Verification items for the finished model (mm, model axes). A direction names the side the tool comes from. Round coordinates to 2 decimals unless told otherwise and drop trailing zeros. Loops run counter-clockwise (first coordinate to the right, second up) from the corner with the lowest first, then second, coordinate; pieces in that order, holes last. Notation, with made-up numbers: M 61.5,44.25 L 76.5,44.25 A33 cw 76.5,72.25 Z; hole C 82.25,27 d10. An arc over 180 degrees is marked long. One line per item, written item: value.
Autodesk Inventor part; units mm, degrees
ref_plane "Work Plane1" through (0, 12.7, 0) normal (0, -1, 0) x (1, 0, 0)
ref_plane "YZ Plane" through (0, 0, 0) normal (1, 0, 0) x (0, 1, 0)
ref_plane "XZ Plane" through (0, 0, 0) normal (0, 1, 0) x (-1, 0, 0)
sketch "Sketch1" plane through (0, 0, 0) normal (0, 0, 1) x (1, 0, 0)
  line L0 (0, 0) -> (50.8, 0)
  line L1 (50.8, 0) -> (50.8, 25.4)
  line L2 (50.8, 25.4) -> (0, 25.4)
  line L3 (0, 25.4) -> (0, 0)
  line L4 (3.175, 22.225) -> (47.625, 22.225)
  line L5 (47.625, 22.225) -> (47.625, 3.175)
  line L6 (47.625, 3.175) -> (3.175, 3.175)
  line L7 (3.175, 3.175) -> (3.175, 22.225)
  dimension "d0" = 50.8
  dimension "d1" = 25.4
  dimension "d2" = 3.175
extrude "Extrusion1" add sketch "Sketch1" along normal blind 152.4
sketch "Sketch2" plane through (0, 25.4, 0) normal (0, 1, 0) x (1, 0, 0)
  line L0 (0, -152.4) -> (50.8, -152.4)
  line L1 (0, 0) -> (0, -152.4)
  circle A0 centre (25.4, -127) radius 3.75
  dimension "d5" = 7.5
  dimension "d6" = 25.4
  dimension "d7" = 25.4
extrude "Extrusion2" cut sketch "Sketch2" against normal blind 76.2
ref_plane "Work Plane1" through (0, 12.7, 0) normal (0, -1, 0) x (1, 0, 0)
properties part number "Spinner brace" material "Aluminum 6061"
(1) Tool access check on faces 1 (the face through (25, 23, 0)), 2 (the face through (3.175, 13, 75)). Record the directions out of +Z, -Z, +X, -X, +Y, -Y that give a thin tool (end or side, any length) a straight path to the whole face; none if there is none.
Completed:
face 1: -Z, +X, -X, +Y, -Y
face 2: +Z, -Z
(2) Sectioned sample at B-B on z = 127. Enter the section's corners in (x, y) (3 decimals).
Completed:
outline: M 0,0 L 21.65,0 L 21.65,3.175 L 3.175,3.175 L 3.175,22.225 L 21.65,22.225 L 21.65,25.4 L 0,25.4 Z; M 29.15,0 L 50.8,0 L 50.8,25.4 L 29.15,25.4 L 29.15,22.225 L 47.625,22.225 L 47.625,3.175 L 29.15,3.175 Z
(3) Thickness scan on L1, parallel to Z at x = 25.4, y = 23.6; L2, parallel to X at y = 17, z = 9.5 (3 decimals); L3, parallel to X at y = 1.6, z = 127. Record the ranges inside material, lowest first. Write a range as from..to.
Completed:
L1: z = 0..123.25, 130.75..152.4
L2: x = 0..3.175, 47.625..50.8
L3: x = 0..21.65, 29.15..50.8
(4) Mould release check, pull along Y, two halves, no side actions. Record for faces 3 (the face through (26, 3.175, 75)), 4 (the face through (26, 25.4, 75)), 5 (the face through (25, 22.225, 75)), 6 (the face through (25, 0, 75)): +Y half, -Y half, draft (parallel to the pull), parting line (faces both ways), or undercut.
Completed:
face 3: undercut
face 4: +Y half
face 5: undercut
face 6: -Y half
(5) Sectioned sample at D-D on x = 25.4. Enter the section's corners in (y, z) (3 decimals), and give its area (3 significant figures).
Completed:
outline: M 0,0 L 3.175,0 L 3.175,123.25 L 0,123.25 Z; M 0,130.75 L 3.175,130.75 L 3.175,152.4 L 0,152.4 Z; M 22.225,0 L 25.4,0 L 25.4,123.25 L 22.225,123.25 Z; M 22.225,130.75 L 25.4,130.75 L 25.4,152.4 L 22.225,152.4 Z
area: 920 mm^2
(6) Sectioned sample at A-A on x = 42. Enter the section's corners in (y, z) (3 decimals), and give its area (3 significant figures).
Completed:
outline: M 0,0 L 3.175,0 L 3.175,152.4 L 0,152.4 Z; M 22.225,0 L 25.4,0 L 25.4,152.4 L 22.225,152.4 Z
area: 968 mm^2
(7) Sectioned sample at C-C on y = 4.5. Enter the section's corners in (x, z) (3 decimals).
Completed:
outline: M 0,0 L 3.175,0 L 3.175,152.4 L 0,152.4 Z; M 47.625,0 L 50.8,0 L 50.8,152.4 L 47.625,152.4 Z
